from build123d import *

# Parameters (mm, degrees)
ESQUISSE1_R        = 4.95
ESQUISSE1_R_2      = 2.55
BOSS_EXTRU_1_DEPTH = 2
ESQUISSE2_R        = 6.05
ESQUISSE2_R_2      = 4.85
BOSS_EXTRU_2_DEPTH = 2.8
CHANFREIN1_SIZE    = 2
CHANFREIN2_SIZE    = 0.4


with BuildPart() as part:
    # Esquisse1 → Boss.-Extru.1 (new body)
    with BuildSketch(Plane.XY):
        Circle(ESQUISSE1_R)
        Circle(ESQUISSE1_R_2, mode=Mode.SUBTRACT)
    extrude(amount=BOSS_EXTRU_1_DEPTH)

    # Esquisse2 → Boss.-Extru.2 (add)
    with BuildSketch(Plane.XY.offset(2)):
        Circle(ESQUISSE2_R)
        Circle(ESQUISSE2_R_2, mode=Mode.SUBTRACT)
    extrude(amount=BOSS_EXTRU_2_DEPTH)

    # Chanfrein1
    # the kernel refuses this chamfer: 2 mm, written as the material it adds along each edge
    with BuildSketch(Plane(origin=(0, 0, 2), x_dir=(1, 0, 0), z_dir=(0, -1, 0))) as chanfrein1_piece_1_section:
        Polygon((4.95, -CHANFREIN1_SIZE), (4.95 + CHANFREIN1_SIZE, 0), (4.95, 0), align=None)
    chanfrein1_piece_1 = revolve(axis=Axis((0, 0, 2), (0, 0, 1)), mode=Mode.PRIVATE)
    chanfrein1_piece_1 = split(chanfrein1_piece_1, bisect_by=Plane(origin=(-5.472506069, 0, 0), z_dir=(0, 0, 1)), keep=Keep.TOP, mode=Mode.PRIVATE)
    chanfrein1_piece_1 = chanfrein1_piece_1 & Plane(origin=(0, 0, 0.577493931), x_dir=(1, 0, 0), z_dir=(0, 0, -1)) * Cylinder(6.05, 28, mode=Mode.PRIVATE)
    add(chanfrein1_piece_1)

    # Chanfrein2
    chanfrein2_edges = [part.edges().sort_by_distance(p)[0] for p in [
        (-4.85, 0, 4.8),
        (-2.55, 0, 0),
    ]]
    chamfer(chanfrein2_edges, length=CHANFREIN2_SIZE)


solid = part.part
Read the model definition and answer for the solid it produces. Units are mm, in the model's axes. A direction names the side the tool comes from. Round coordinates to 2 decimals unless told otherwise and drop trailing zeros. Write each loop counter-clockwise with the first axis right and the second up, starting at its lowest first coordinate (ties: lowest second). Pieces come first, ordered by that corner, then holes.
1. Determine the mould class of faces 3 (the face through (3.2, 0.1, 0)), 4 (the face through (5.589, 2.317, 2.924)), 5 (the face through (1.18, -2.26, 1.19)) for opening direction Y: pulls with the +Y half, pulls with the -Y half, needs draft (parallel to the pull), parting line crosses it, or undercut.
2. Which of the six approach directions +Z, -Z, +X, -X, +Y, -Y give full straight-line access (tool end or side, diameter ignored) to faces 1 (the face through (4.626, 1.457, 3.183)), 2 (the face through (-5, 3, 4.8))?
3. The part is cut by section C-C, the plane z = 0.6. Determine the outline of the cut face in (x, y), then the cut area to 3 significant figures.
4. The part is cut by section D-D, the plane z = 1.3. Determine the outline of the cut face in (x, y), then the cut area to 3 significant figures.
5. The part is cut by section A-A, the plane y = 0. Determine the outline of the cut face in (x, z).
6. Given pin 1 Ø2 at (y, z) = (-3, 2) entering from -X; pin 2 Ø4 at (x, y) = (0, 0) entering from +Z; pin 3 Ø5 at (x, y) = (-2.5, 0) entering from +Z; pin 4 Ø1.5 at (x, z) = (4.5, 1) entering from +Y, each flat-ended and moving along its own axis, determine where each tip first touches the part or whether it passes through.
7. Straight lines are drawn through the part: L1, parallel to Y at x = 0, z = 3.15; L2, parallel to Z at x = -3.25, y = -1.75; L3, parallel to X at y = 2, z = 2.1. For each, find the intervals that lie inside material, in ascending order.
Values:
1. face 3: needs draft
1. face 4: parting line crosses it
1. face 5: undercut
2. face 1: +Z
2. face 2: +Z, +X, -X, +Y, -Y
3. outline: circle Ø11.1 at (0, 0); hole circle Ø5.1 at (0, 0)
3. area: 76.3 mm2
4. outline: circle Ø12.1 at (0, 0); hole circle Ø5.1 at (0, 0)
4. area: 94.6 mm2
5. outline: (-6.05, 1.1) - (-4.95, 0) - (-2.95, 0) - (-2.55, 0.4) - (-2.55, 2) - (-4.85, 2) - (-4.85, 4.4) - (-5.25, 4.8) - (-6.05, 4.8) - close; (2.55, 0.4) - (2.95, 0) - (4.95, 0) - (6.05, 1.1) - (6.05, 4.8) - (5.25, 4.8) - (4.85, 4.4) - (4.85, 2) - (2.55, 2) - close
6. pin 1: stops at x = -5.71
6. pin 2: passes through
6. pin 3: stops at z = 4.55
6. pin 4: stops at y = 4.74
7. L1: y = -6.05 to -4.85, 4.85 to 6.05
7. L2: z = 0 to 2
7. L3: x = -5.71 to -4.42, 4.42 to 5.71
